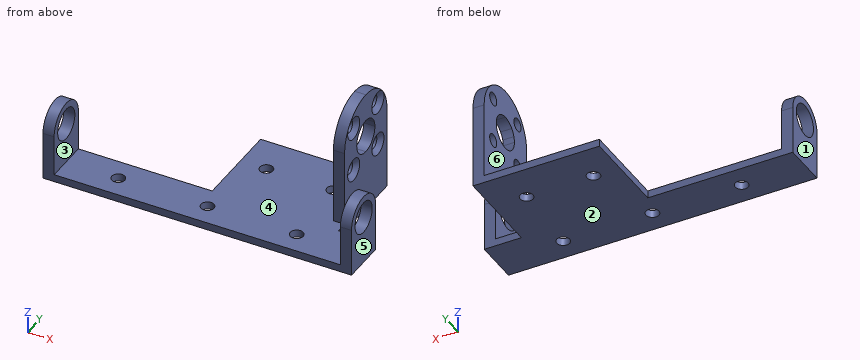
from build123d import *

# Parameters (mm, degrees)
F0_R            = 1.75
F1_DEPTH        = 2
F3_R            = 4.25
F4_DEPTH        = 3
F5_R            = 4.25
F6_DEPTH        = 3
F9_DEPTH        = 3
F10_D           = 3.5
F10_CSINK_D     = 6
F10_CSINK_ANGLE = 90


with BuildPart() as f1:
    # F0 (on Top) → F1 (new body)
    with BuildSketch(Plane.XY):
        Polygon((0, 12), (0, 0), (83, 0), (83, 12), (73, 12), (73, 36), (39, 36), (39, 12), align=None)
        with Locations((17, 6)):
            Circle(F0_R, mode=Mode.SUBTRACT)
        with Locations((41, 6)):
            Circle(F0_R, mode=Mode.SUBTRACT)
        with Locations((65, 6)):
            Circle(F0_R, mode=Mode.SUBTRACT)
        with Locations((46, 26)):
            Circle(F0_R, mode=Mode.SUBTRACT)
        with Locations((64, 26)):
            Circle(F0_R, mode=Mode.SUBTRACT)
    extrude(amount=F1_DEPTH)

    # F3 (on Right) → F4 (join)
    with BuildSketch(Plane.YZ):
        with BuildLine():
            Line((0, 13), (0, 0))
            Line((0, 0), (12, 0))
            Line((12, 0), (12, 13))
            ThreePointArc((12, 13), (6, 19), (0, 13))
        make_face()
        with Locations((6, 13)):
            Circle(F3_R, mode=Mode.SUBTRACT)
    extrude(amount=F4_DEPTH)

    # F5 (on offset) → F6 (join)
    with BuildSketch(Plane.YZ.offset(83)):
        with BuildLine():
            Line((0, 13), (0, 0))
            Line((0, 0), (12, 0))
            Line((12, 0), (12, 13))
            ThreePointArc((12, 13), (6, 19), (0, 13))
        make_face()
        with Locations((6, 13)):
            Circle(F5_R, mode=Mode.SUBTRACT)
    extrude(amount=-F6_DEPTH)

    # F8 (on offset) → F9 (join)
    with BuildSketch(Plane.YZ.offset(73)):
        with BuildLine():
            Line((15, 22.5), (15, 0))
            Line((15, 0), (36, 0))
            Line((36, 0), (36, 22.5))
            Line((36, 22.5), (29.742641, 22.5))
            ThreePointArc((29.742641, 22.5), (29.935194, 21.760959), (30, 21))
            ThreePointArc((30, 21), (28.681981, 17.818019), (25.5, 16.5))
            ThreePointArc((25.5, 16.5), (22.318019, 17.818019), (21, 21))
            ThreePointArc((21, 21), (21.064806, 21.760959), (21.257359, 22.5))
            Line((21.257359, 22.5), (15, 22.5))
        make_face()
        with BuildLine():
            ThreePointArc((25.5, 33), (18.075379, 29.924621), (15, 22.5))
            Line((15, 22.5), (21.257359, 22.5))
            ThreePointArc((21.257359, 22.5), (21.693622, 23.400309), (22.318019, 24.181981))
            ThreePointArc((22.318019, 24.181981), (23.777925, 25.157458), (25.5, 25.5))
            Line((25.5, 25.5), (25.5, 33))
        make_face()
        with BuildLine():
            Line((29.742641, 22.5), (36, 22.5))
            ThreePointArc((36, 22.5), (32.924621, 29.924621), (25.5, 33))
            Line((25.5, 33), (25.5, 25.5))
            ThreePointArc((25.5, 25.5), (28.098076, 24.674235), (29.742641, 22.5))
        make_face()
    extrude(amount=-F9_DEPTH)

    # F10 (through all)
    with Locations(Plane.YZ.offset(73)):
        with Locations((31.510408, 14.989592), (19.489592, 14.989592), (19.489592, 27.010408), (31.510408, 27.010408)):
            CounterSinkHole(F10_D / 2, F10_CSINK_D / 2, counter_sink_angle=F10_CSINK_ANGLE)


solid = f1.part
The listing builds one solid part. Answer for the finished solid, in the listing's coordinates (mm). Face numbers are marked on the shaded views. A direction names the side the tool comes from. Round coordinates to 2 decimals unless told otherwise and drop trailing zeros. Write each loop counter-clockwise with the first axis right and the second up, starting at its lowest first coordinate (ties: lowest second). Pieces come first, ordered by that corner, then holes. Notation, with made-up numbers: (47.5, 52.25) - (87.5, 52.25) arc R32 cw to (87.5, 89.25) - close; hole circle Ø6 at (-5.75, 72.25). An arc over 180 degrees is marked (long way). Use a Markdown table: item, result. Add a question column.
1. The part is cut by section A-A (x = 17). Write down the section's boundary in (y, z), and give its area (3 significant figures).
2. Flat-ended cylindrical pins translate along their axes: P1, Ø10, axis at y = 25, z = 7.5, coming from the -X side; P2, Ø1.6, axis at y = 22.5, z = 0.5, coming from the -X side; P3, Ø8, axis at x = 60.5, y = 30.5, coming from the +Z side; P4, Ø3, axis at x = 41, y = 6, coming from the +Z side. Find the tip coordinate at first contact, or state that the pin passes through.
3. A tool of negligible diameter and unlimited length cuts with its end or side. For the marked faces 5 and 6, from which of +Z, -Z, +X, -X, +Y, -Y can it reach the whole face along a straight path? Write none if from no direction.
4. The part is cut by section B-B (y = 3). Write down the section's boundary in (x, z).
5. For a pull along X with two mould halves and no side action, classify the marked faces 1, 2, 3 and 4 as +X half, -X half, draft (parallel to the pull), parting line (faces both ways), or undercut.
6. Consider line 1 (X direction, y = 2.5, z = 10.5); line 2 (Z direction, x = 0.75, y = 6); line 3 (Z direction, x = 43, y = 18). Determine where each line is inside the solid, lowest interval first.
7. The part is cut by section C-C (x = 41). Write down the section's boundary in (y, z).
Reported:
| question | item | result |
|---|---|---|
| 1 | outline | (0, 0) - (4.25, 0) - (4.25, 2) - (0, 2) - close; (7.75, 0) - (12, 0) - (12, 2) - (7.75, 2) - close |
| 1 | area | 17.0 mm^2 |
| 2 | P1 | x = 70 |
| 2 | P2 | x = 39 |
| 2 | P3 | z = 2 |
| 2 | P4 | through |
| 3 | face 5 | +Z, -Z, +X, +Y, -Y |
| 3 | face 6 | +Z, -X, +Y, -Y |
| 4 | outline | (0, 0) - (83, 0) - (83, 9.99) - (80, 9.99) - (80, 2) - (3, 2) - (3, 9.99) - (0, 9.99) - close; (0, 16.01) - (3, 16.01) - (3, 18.2) - (0, 18.2) - close; (80, 16.01) - (83, 16.01) - (83, 18.2) - (80, 18.2) - close |
| 5 | face 1 | -X half |
| 5 | face 2 | draft |
| 5 | face 3 | undercut |
| 5 | face 4 | undercut |
| 6 | line 1 | 0 to 3, 80 to 83 |
| 6 | line 2 | 0 to 8.75, 17.25 to 19 |
| 6 | line 3 | 0 to 2 |
| 7 | outline | (0, 0) - (4.25, 0) - (4.25, 2) - (0, 2) - close; (7.75, 0) - (36, 0) - (36, 2) - (7.75, 2) - close |
